Autodesk Inventor part; units mm, degrees
ref_plane "YZ Plane" through (0, 0, 0) normal (1, 0, 0) x (0, 1, 0)
ref_plane "XZ Plane" through (0, 0, 0) normal (0, 1, 0) x (-1, 0, 0)
ref_plane "XY Plane" through (0, 0, 0) normal (0, 0, 1) x (1, 0, 0)
sketch "スケッチ1" plane through (0, 0, 0) normal (0, 1, 0) x (-1, 0, 0)
  line L0 (20, 22) -> (-20, 22)
  line L1 (-20, 22) -> (-20, -22)
  line L2 (-20, -22) -> (20, -22)
  line L3 (20, -22) -> (20, 22)
  line L4 (20, 22) -> (-20, -22) construction
  line L5 (-20, 22) -> (20, -22) construction
  point P0 (0, 0)
  dimension "d0" = 40
  dimension "d1" = 44
extrude "押し出し1" add sketch "スケッチ1" along normal blind 40
sketch "スケッチ2" plane through (0, 40, 0) normal (0, 1, 0) x (1, 0, 0)
  line L0 (-20, -20) -> (20, -20)
  line L1 (20, -20) -> (20, 20)
  line L2 (20, 20) -> (-20, 20)
  line L3 (-20, 20) -> (-20, -20)
  line L4 (-20, -20) -> (20, 20) construction
  line L5 (20, -20) -> (-20, 20) construction
  point P0 (0, 0)
  dimension "d4" = 40
  dimension "d5" = 40
extrude "押し出し2" cut sketch "スケッチ2" against normal blind 38
sketch "スケッチ3" plane through (0, 0, 0) normal (0, -1, 0) x (1, 0, 0)
  line L0 (-20, -22) -> (-20, 22)
  line L1 (-20, 22) -> (20, 22)
  point P0 (0, 0)
  point P1 (-10, 10)
  point P2 (10, 10)
  point P3 (-10, -10)
  point P4 (10, -10)
  dimension "d8" = 10
  dimension "d9" = 12
  dimension "d12" = 20
  dimension "d15" = 20
hole "穴1" at (-10, 0, 10) at (10, 0, 10) at (-10, 0, -10) at (10, 0, -10) direction (0, 1, 0) diameter 4 end through all
sketch "スケッチ4" plane through (-20, 0, 22) normal (0, 0, 1) x (1, 0, 0)
  line L0 (0, 0) -> (0, 40)
  point P0 (20, 0)
  point P1 (20, 35)
  dimension "d25" = 35
  dimension "d26" = 20
hole "穴2" at (0, 35, 22) direction (0, 0, -1) diameter 4 end through all
properties part number "blaket_2"
Model file for the job. Use its own axes, mm. A direction names the side the tool comes from. Give positions to 0.01 mm unless a question says otherwise; leave off trailing zeros. Order: outer loops, then holes, each group sorted by start corner. A loop starts at its lowest first (then second) coordinate and runs counter-clockwise, first axis right, second up. Notation, with made-up numbers: M 48.25,-28.75 L 101.25,-28.75 A20 cw 101.25,4.25 Z; hole C 4,35 d11. An arc over 180 degrees is marked long. Put each result on its own line as item: value. Start each with the question number.
(1) Band-saw the part on B-B on y = 11. Give the cut face in (x, z), then the cut area to 3 significant figures.
(2) Pin check, flat tips, straight feed: pin 1 Ø4 at (x, z) = (11.5, -3.5) entering from +Y; pin 2 Ø3 at (x, y) = (0, 35) entering from +Z. Stop position of each tip, or through.
(3) Drill centre lines: L1, parallel to X at y = 0.4, z = -10; L2, parallel to Z at x = 10, y = 1; L3, parallel to Z at x = -9.5, y = 7. Where is each one in solid material? Low to high. Write a range as [from, to].
(4) Band-saw the part on C-C on x = -10. Give the cut face in (y, z).
(5) Pull direction Z, two halves, no side cores. Call faces 3 (the face through (0, 21, -20)), 4 (the face through (0.766, 33.153, -21.014)), 5 (the face through (0, 20, -22)): released by +Z, released by -Z, zero draft, split by the parting line, or undercut.
(6) Tool access for faces 1 (the face through (0, 2, 0)), 2 (the face through (0, 20, 22)): list every direction of +Z, -Z, +X, -X, +Y, -Y with a clear straight run to the whole face (end or side of a thin tool).
(7) Band-saw the part on A-A on z = 10. Give the cut face in (x, y), then the cut area to 3 significant figures.
(8) Band-saw the part on D-D on y = 35. Give the cut face in (x, z).
Results below:
1. outline: M -20,-22 L 20,-22 L 20,-20 L -20,-20 Z; M -20,20 L 20,20 L 20,22 L -20,22 Z
1. area: 160 mm2
2. pin 1: stops at y = 2
2. pin 2: passes through
3. L1: x = [-20, -12], [-8, 8], [12, 20]
3. L2: z = [-22, -12], [-8, 8], [12, 22]
3. L3: z = [-22, -20], [20, 22]
4. outline: M 0,-22 L 40,-22 L 40,-20 L 2,-20 L 2,-12 L 0,-12 Z; M 0,-8 L 2,-8 L 2,8 L 0,8 Z; M 0,12 L 2,12 L 2,20 L 40,20 L 40,22 L 0,22 Z
5. face 3: undercut
5. face 4: zero draft
5. face 5: released by -Z
6. face 1: +X, -X, +Y
6. face 2: +Z, +X, -X, +Y, -Y
7. outline: M -20,0 L -12,0 L -12,2 L -20,2 Z; M -8,0 L 8,0 L 8,2 L -8,2 Z; M 12,0 L 20,0 L 20,2 L 12,2 Z
7. area: 64.0 mm2
8. outline: M -20,-22 L -2,-22 L -2,-20 L -20,-20 Z; M -20,20 L -2,20 L -2,22 L -20,22 Z; M 2,-22 L 20,-22 L 20,-20 L 2,-20 Z; M 2,20 L 20,20 L 20,22 L 2,22 Z
